from build123d import *

# Parameters (mm, degrees)
PAD031_DEPTH            = 3.75
SKETCH061_R             = 1.5
POCKET029_DEPTH         = 3.75
POCKET035_DEPTH         = 2
SKETCH063_R             = 1.5
POCKET036_DEPTH         = 1.3
SKETCH064_R             = 2.2
PAD037_DEPTH            = 3
SKETCH065_W             = 2.8
SKETCH065_H             = 4
PAD038_DEPTH            = 2
SKETCH066_R             = 0.75
POCKET037_DEPTH         = 3
FILLET022_R             = 0.99
SKETCH073_W             = 2.2
SKETCH073_H             = 5
POCKET040_DEPTH         = 0.5
PAD197_DEPTH            = 0.4
PAD197_FACE23_W         = 5
PAD197_FACE23_H         = 2.5
PAD198_DEPTH            = 0.25
SKETCH338_R             = 1.55
SKETCH338_R_2           = 1.5
POCKET161_DEPTH         = 5
PAD201_DEPTH            = 2
PAD202_DEPTH            = 1
BODY006_ROLL_ANGLE      = -90
BODY006_PLACEMENT_ANGLE = -90


with BuildPart() as part:
    # Sketch060 → Pad031 (new body)
    with BuildSketch(Plane(origin=(-1, 0, -1.2), x_dir=(1, 0, 0), z_dir=(0, 0, 1))):
        with BuildLine():
            ThreePointArc((0, -3), (3, 0), (0, 3))
            Line((0, 3), (-3.2, 3))
            Line((-3.2, 3), (-3.2, 4))
            Line((-3.2, 4), (-12.7, 4))
            Line((-12.7, -4), (-12.7, 4))
            Line((-3.2, -4), (-12.7, -4))
            Line((-3.2, -3), (-3.2, -4))
            Line((0, -3), (-3.2, -3))
        make_face()
    extrude(amount=PAD031_DEPTH)

    # Sketch061 (on Face10 of Pad031) → Pocket029 (cut)
    with BuildSketch(Plane.XY.offset(2.55)):
        with Locations((-1, 0)):
            Circle(SKETCH061_R)
    extrude(amount=-POCKET029_DEPTH, mode=Mode.SUBTRACT)

    # Sketch062 (on DatumPlane) → Pocket035 (cut)
    with BuildSketch(Plane.XY.offset(2.55)):
        with BuildLine():
            ThreePointArc((-1, -2), (1, 0), (-1, 2))
            Line((-1, 2), (-10.2, 2))
            Line((-10.2, 2), (-10.2, 2.5))
            Line((-10.2, 2.5), (-12.4, 2.5))
            Line((-12.4, -2.5), (-12.4, 2.5))
            Line((-10.2, -2.5), (-12.4, -2.5))
            Line((-10.2, -2), (-10.2, -2.5))
            Line((-1, -2), (-10.2, -2))
        make_face()
    extrude(amount=-POCKET035_DEPTH, mode=Mode.SUBTRACT)

    # Sketch063 (on DatumPlane) → Pocket036 (cut)
    with BuildSketch(Plane(origin=(-13.7, 0, 0), x_dir=(0, -1, 0), z_dir=(-1, 0, 0))):
        with Locations((0, 2.511938)):
            Circle(SKETCH063_R)
    extrude(amount=-POCKET036_DEPTH, mode=Mode.SUBTRACT)

    # Sketch064 (on DatumPlane) → Pad037 (join)
    with BuildSketch(Plane.XY.offset(0.55)):
        with Locations((-7.35, 0)):
            Circle(SKETCH064_R)
    extrude(amount=PAD037_DEPTH)

    # Sketch065 (on DatumPlane) → Pad038 (join)
    with BuildSketch(Plane.XY.offset(0.55)):
        with Locations((-8.8, 0)):
            Rectangle(SKETCH065_W, SKETCH065_H)
    extrude(amount=PAD038_DEPTH)

    # Sketch066 (on DatumPlane) → Pocket037 (cut)
    with BuildSketch(Plane.XY.offset(3.55)):
        with Locations((-7.35, 0)):
            Circle(SKETCH066_R)
    extrude(amount=-POCKET037_DEPTH, mode=Mode.SUBTRACT)

    # Fillet022
    fillet022_edges = [part.edges().sort_by_distance(p)[0] for p in [
        (-4.2, 4, 0.675),
        (-4.2, -4, 0.675),
    ]]
    fillet(fillet022_edges, radius=FILLET022_R)

    # Sketch073 (on DatumPlane) → Pocket040 (cut)
    with BuildSketch(Plane.XY.offset(0.55)):
        with Locations((-11.3, 0)):
            Rectangle(SKETCH073_W, SKETCH073_H)
    extrude(amount=-POCKET040_DEPTH, mode=Mode.SUBTRACT)

    # Pocket040 Face23 → Pad197 (add)
    with BuildSketch(Plane(origin=(-12.4, 0, 1.054406), x_dir=(0, -1, 0), z_dir=(1, 0, 0))):
        with BuildLine():
            Line((1.499517, -1.495594), (2.5, -1.495594))
            Line((2.5, -1.495594), (2.5, 1.004406))
            Line((2.5, 1.004406), (-2.5, 1.004406))
            Line((-2.5, 1.004406), (-2.5, -1.495594))
            Line((-2.5, -1.495594), (-1.499517, -1.495594))
            ThreePointArc((-1.499517, -1.495594), (-0.019033, 0.042347), (1.5, -1.457532))
            ThreePointArc((1.5, -1.457532), (1.499879, -1.476565), (1.499517, -1.495594))
        make_face()
    extrude(amount=PAD197_DEPTH)

    # Pad197 Face23 → Pad198 (add)
    with BuildSketch(Plane(origin=(-10.2, 0, 1.3), x_dir=(0, 1, 0), z_dir=(-1, 0, 0))):
        Rectangle(PAD197_FACE23_W, PAD197_FACE23_H)
    extrude(amount=PAD198_DEPTH)

    # Sketch338 (on Face18 of Pad198) → Pocket161 (cut)
    with BuildSketch(Plane.XY.offset(0.55)):
        with Locations((-1, 0)):
            Circle(SKETCH338_R)
        with Locations((-1, 0)):
            Circle(SKETCH338_R_2, mode=Mode.SUBTRACT)
    extrude(amount=-POCKET161_DEPTH, mode=Mode.SUBTRACT)

    # Sketch339 (on Face23 of Pocket161) → Pad201 (join)
    with BuildSketch(Plane.XY.offset(0.55)):
        with BuildLine():
            ThreePointArc((-0.5, 1.46714), (-1, 1.55), (-1.5, 1.46714))
            Line((-1.5, 1.936492), (-1.5, 1.46714))
            ThreePointArc((-0.5, 1.936492), (-1, 2), (-1.5, 1.936492))
            Line((-0.5, 1.936492), (-0.5, 1.46714))
        make_face()
        with BuildLine():
            ThreePointArc((-1.5, -1.46714), (-1, -1.55), (-0.5, -1.46714))
            Line((-0.5, -1.46714), (-0.5, -1.936492))
            ThreePointArc((-1.5, -1.936492), (-1, -2), (-0.5, -1.936492))
            Line((-1.5, -1.46714), (-1.5, -1.936492))
        make_face()
        with BuildLine():
            ThreePointArc((-2.46714, 0.5), (-2.55, 0), (-2.46714, -0.5))
            Line((-2.46714, -0.5), (-2.936492, -0.5))
            ThreePointArc((-2.936492, 0.5), (-3, 0), (-2.936492, -0.5))
            Line((-2.46714, 0.5), (-2.936492, 0.5))
        make_face()
        with BuildLine():
            ThreePointArc((0.46714, -0.5), (0.55, 0), (0.46714, 0.5))
            Line((0.936492, 0.5), (0.46714, 0.5))
            ThreePointArc((0.936492, -0.5), (1, 0), (0.936492, 0.5))
            Line((0.936492, -0.5), (0.46714, -0.5))
        make_face()
    extrude(amount=PAD201_DEPTH)

    # Sketch340 (on Face31 of Pad201) → Pad202 (join)
    with BuildSketch(Plane.XY.offset(2.55)):
        with BuildLine():
            ThreePointArc((-2.46714, 0.5), (-2.55, 0), (-2.46714, -0.5))
            Line((-2.414214, -0.5), (-2.46714, -0.5))
            ThreePointArc((-2.414214, 0.5), (-2.5, 0), (-2.414214, -0.5))
            Line((-2.414214, 0.5), (-2.46714, 0.5))
        make_face()
        with BuildLine():
            ThreePointArc((-1.5, -1.46714), (-1, -1.55), (-0.5, -1.46714))
            Line((-0.5, -1.46714), (-0.5, -1.414214))
            ThreePointArc((-1.5, -1.414214), (-1, -1.5), (-0.5, -1.414214))
            Line((-1.5, -1.46714), (-1.5, -1.414214))
        make_face()
        with BuildLine():
            ThreePointArc((-0.5, 1.46714), (-1, 1.55), (-1.5, 1.46714))
            Line((-1.5, 1.46714), (-1.5, 1.414214))
            ThreePointArc((-0.5, 1.414214), (-1, 1.5), (-1.5, 1.414214))
            Line((-0.5, 1.46714), (-0.5, 1.414214))
        make_face()
        with BuildLine():
            ThreePointArc((0.46714, -0.5), (0.55, 0), (0.46714, 0.5))
            Line((0.414214, 0.5), (0.46714, 0.5))
            ThreePointArc((0.414214, -0.5), (0.5, 0), (0.414214, 0.5))
            Line((0.46714, -0.5), (0.414214, -0.5))
        make_face()
    extrude(amount=-PAD202_DEPTH)


with BuildPart() as part_1:
    # Body006 roll: moved
    add(part.part.rotate(Axis((0, 0, 0), (1, 0, 0)), BODY006_ROLL_ANGLE))


with BuildPart() as part_2:
    # Body006 placement: moved
    add(part_1.part.moved(Location((30.25, -34.7, 7.25))).rotate(Axis((30.25, -34.7, 7.25), (0, 0, 1)), BODY006_PLACEMENT_ANGLE))


solid = part_2.part
Design review of the part built by this model. Coordinates are the model's own, in mm. A direction names the side the tool comes from. Give positions to 0.01 mm unless a question says otherwise; leave off trailing zeros. Order: outer loops, then holes, each group sorted by start corner. A loop starts at its lowest first (then second) coordinate and runs counter-clockwise, first axis right, second up. Notation, with made-up numbers: (-37.75, 28) - (18.25, 28) arc R31 ccw to (18.25, 54) - close; hole circle Ø7 at (-15.5, 19.5). An arc over 180 degrees is marked (long way). Use CSV: the item, a comma, the result in double quotes. Start each with the question number.
Q1. Machinability: for faces 1 (the face through (32, -24.25, 7)), 2 (the face through (31, -32, 10.25)), 3 (the face through (32.3, -35.2, 7.3)), which of the approach directions +Z, -Z, +X, -X, +Y, -Y give a long, thin tool a straight path to every point of the face, cutting with its end or side? Answer none if there is none.
Q2. For P1, Ø0.6, axis at x = 31.5, y = -30, coming from the +Z side; P2, Ø1.2, axis at y = -23.5, z = 7.5, coming from the +X side; P3, Ø0.8, axis at x = 31, z = 6.5, coming from the -Y side, all flat-tipped, find the tip position at first contact; note any pin that passes through.
Q3. Take a section at B-B (y = -33). State the section outline as (x, z) points.
Q4. Take a section at C-C (x = 31.1). Count the separate pieces of the cut face and the enclosed holes in it, and give its area (3 significant figures).
Q5. Draft analysis for pull direction Y (two halves, no side actions). For faces 4 (the face through (31, -25, 3.25)), 5 (the face through (32.3, -32.2, 7.2)), 6 (the face through (30.95, -30.22, 3.55)), 7 (the face through (30.8, -34.9, 8.5)), state which applies: pulls with the +Y half, pulls with the -Y half, needs draft (parallel to the pull), parting line crosses it, or undercut.
Q6. For line 1 (Y direction, x = 31.9, z = 7.25); line 2 (Z direction, x = 32.05, y = -27.35); line 3 (Y direction, x = 31.4, z = 8.5), list the stretches that pass through material, from the lowest coordinate up.
Q7. Take a section at A-A (z = 7.25). State the section outline as (x, y) points.
Q8. Take a section at D-D (y = -23.5). State the section outline as (x, z) points, and give its area (3 significant figures).
Calculated:
1,face 1,"+X"
1,face 2,"+Z, +X, -X, -Y"
1,face 3,"+X, -X"
2,P1,"stops at z = 11.23"
2,P2,"stops at x = 30.3"
2,P3,"stops at y = -36.68"
3,outline,"(29.05, 4.25) - (32.8, 4.25) - (32.8, 5.25) - (30.8, 5.25) - (30.8, 5.87) - (29.05, 5.87) - close; (29.05, 8.63) - (30.8, 8.63) - (30.8, 9.25) - (32.8, 9.25) - (32.8, 10.25) - (29.05, 10.25) - close"
4,separate pieces,"2"
4,enclosed holes,"3"
4,area,"76.9 mm²"
5,face 4,"needs draft"
5,face 5,"undercut"
5,face 6,"pulls with the -Y half"
5,face 7,"undercut"
6,line 1,"y = -36.7 to -35.2, -32.2 to -31.7, -29.55 to -28.1, -26.6 to -24.25"
6,line 2,"z = 3.25 to 6.5, 8 to 11.25"
6,line 3,"y = -36.43 to -35.26, -29.16 to -24.25, -22.7 to -21"
7,outline,"(29.05, -36.7) - (32.8, -36.7) - (32.8, -35.2) - (31.8, -35.2) - (31.8, -35.25) - (29.05, -35.25) - close; (29.05, -32.15) - (31.8, -32.15) - (31.8, -32.2) - (32.8, -32.2) - (32.8, -31.7) - (30.8, -31.7) - (30.8, -29.55) - (33.8, -29.55) - (33.8, -28.1) - (30.8, -28.1) - (30.8, -26.6) - (33.8, -26.6) - (33.8, -25.15) - (32.8, -25.15) - (32.8, -24.25) - (30.3, -24.25) - (30.3, -22.7) - (31.26, -22.7) - (31.26, -21) - (29.05, -21) - close"
8,outline,"(29.05, 3.25) - (32.8, 3.25) - (32.8, 4.75) - (30.3, 4.75) - (30.3, 9.75) - (32.8, 9.75) - (32.8, 11.25) - (29.05, 11.25) - close"
8,area,"17.5 mm²"
